The model under review builds one solid part; all positions refer to its coordinate system, in mm. Face numbers are marked on the shaded views. A direction names the side the tool comes from. Coordinates: 2 decimals unless noted, no trailing zeros. Order: outer loops, then holes, each group sorted by start corner. A loop starts at its lowest first (then second) coordinate and runs counter-clockwise, first axis right, second up.
```python
from build123d import *

# Parameters (mm, degrees)
F0_W      = 29
F0_H      = 29
F1_DEPTH  = 42
F2_R      = 14.5
F2_R_2    = 13.5
F3_DEPTH  = 12
F4_W      = 34
F4_H      = 25
F5_DEPTH  = 0.1
F6_W      = 34
F6_H      = 25
F7_DEPTH  = 0.1
F8_W      = 28.9
F8_H      = 34
F9_DEPTH  = 0.1
F11_D     = 3.3
F11_DEPTH = 3
F11_TIP   = 0.9914200214
F13_D     = 2.3
F13_DEPTH = 3
F13_TIP   = 0.6909897119
F14_R     = 6.6
F15_DEPTH = 0.5
F16_W     = 12
F16_H     = 10
F17_DEPTH = 0.5
F19_DEPTH = 10
F20_R     = 5
F20_R_2   = 4.2771578829
F21_DEPTH = 5.8


with BuildPart() as f1:
    # F0 (on Front) → F1 (new body)
    with BuildSketch(Plane.XZ):
        Rectangle(F0_W, F0_H)
    extrude(amount=F1_DEPTH)

    # F2 (on face) → F3 (join)
    with BuildSketch(Plane.XZ.offset(42)):
        Circle(F2_R)
        Circle(F2_R_2, mode=Mode.SUBTRACT)
    extrude(amount=F3_DEPTH)

    # F4 (on face) → F5 (cut)
    with BuildSketch(Plane.YZ.offset(14.5)):
        with Locations((-21, 2)):
            Rectangle(F4_W, F4_H)
    extrude(amount=-F5_DEPTH, mode=Mode.SUBTRACT)

    # F6 (on face) → F7 (cut)
    with BuildSketch(Plane(origin=(-14.5, 0, 0), x_dir=(0, -1, 0), z_dir=(-1, 0, 0))):
        with Locations((21, 2)):
            Rectangle(F6_W, F6_H)
    extrude(amount=-F7_DEPTH, mode=Mode.SUBTRACT)

    # F8 (on face) → F9 (cut)
    with BuildSketch(Plane.XY.offset(14.5)):
        with Locations((0.05, -21)):
            Rectangle(F8_W, F8_H)
    extrude(amount=-F9_DEPTH, mode=Mode.SUBTRACT)

    # F11
    with Locations(Plane(origin=(0, 0, -14.5), x_dir=(1, 0, 0), z_dir=(0, 0, -1))):
        with Locations((0, 15.3), (10, 39), (-10, 39)):
            Hole(F11_D / 2, depth=F11_DEPTH)
            with Locations((0, 0, -(F11_DEPTH + F11_TIP / 2))):  # 118° drill point
                Cone(0, F11_D / 2, F11_TIP, mode=Mode.SUBTRACT)

    # F13
    with Locations(Plane(origin=(0, 0, -14.5), x_dir=(1, 0, 0), z_dir=(0, 0, -1))):
        with Locations((6, 15.5), (-6, 15.5), (6, 37.5), (-6, 37.5)):
            Hole(F13_D / 2, depth=F13_DEPTH)
            with Locations((0, 0, -(F13_DEPTH + F13_TIP / 2))):  # 118° drill point
                Cone(0, F13_D / 2, F13_TIP, mode=Mode.SUBTRACT)

    # F14 (on face) → F15 (join)
    with BuildSketch(Plane(origin=(0, 0, 0), x_dir=(-1, 0, 0), z_dir=(0, 1, 0))):
        with Locations((-7.9, -6.2)):
            Circle(F14_R)
    extrude(amount=F15_DEPTH)

    # F16 (on face) → F17 (cut)
    with BuildSketch(Plane(origin=(0, 0, 0), x_dir=(-1, 0, 0), z_dir=(0, 1, 0))):
        with Locations((2.2, 8.5)):
            Rectangle(F16_W, F16_H)
    extrude(amount=-F17_DEPTH, mode=Mode.SUBTRACT)

    # F18 (on face) → F19 (cut)
    with BuildSketch(Plane(origin=(0, -0.5, 0), x_dir=(-1, 0, 0), z_dir=(0, 1, 0))):
        Polygon((-3.1485289801, 10.3262867779), (-3.1485289801, 4.1849459521), (7.6598110609, 4.1849459521), (7.6598110609, 10.3262867779), (5.341138225, 10.3262867779), (5.341138225, 11.5245990455), (4.3890266679, 11.5245990455), (4.3890266679, 12.9305869341), (0, 12.9305869341), (0, 11.5245990455), (-1.0954904137, 11.5245990455), (-1.0954904137, 10.3262867779), align=None)
    extrude(amount=-F19_DEPTH, mode=Mode.SUBTRACT)

    # F20 (on face) → F21 (join)
    with BuildSketch(Plane(origin=(0, 0.5, 0), x_dir=(-1, 0, 0), z_dir=(0, 1, 0))):
        with Locations((-7.9, -6.2)):
            Circle(F20_R)
        with Locations((-7.9, -6.2)):
            Circle(F20_R_2, mode=Mode.SUBTRACT)
    extrude(amount=F21_DEPTH)


solid = f1.part
```
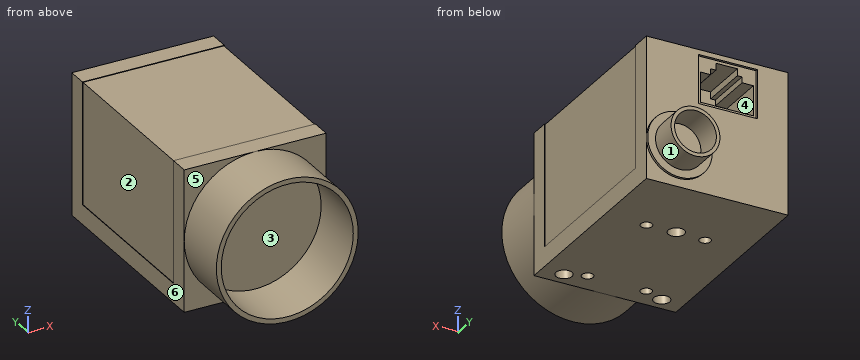
(1) Wall thickness on probe 1 along Y at (x, z) = (6, -12.4); probe 2 along Y at (x, z) = (6, -12.95); probe 3 along X at (y, z) = (-15.3, -12.25): over which ranges is each line inside the solid? List them lowest first.
A:
probe 1: y = -54 to -38.65, -36.35 to -16.65, -14.35 to 0.5
probe 2: y = -54 to -38.65, -36.35 to -16.65, -14.35 to 0
probe 3: x = -14.5 to -7.13, -4.87 to -1.65, 1.65 to 4.87, 7.13 to 14.5
(2) For pin 1 Ø4.5 at (x, z) = (6, 6) entering from -Y; pin 2 Ø10.5 at (x, z) = (5, -8.5) entering from +Y; pin 3 Ø1 at (x, z) = (-10, -5) entering from +Y; pin 4 Ø3 at (x, y) = (6, -15.5) entering from +Z, all flat-tipped, find the tip position at first contact; note any pin that passes through.
A:
pin 1: stops at y = -42
pin 2: stops at y = 6.3
pin 3: stops at y = 0
pin 4: stops at z = 14.4
(3) Draft analysis for pull direction X (two halves, no side actions). For the marked faces 4, 5 and 6, state which applies: released by +X, released by -X, zero draft, split by the parting line, or undercut.
A:
face 4: undercut
face 5: zero draft
face 6: released by -X
(4) We need section B-B, the plane y = -45.5. Write out the cut boundary in (x, z), and give its area (3 significant figures).
A:
outline: circle Ø29 at (0, 0); hole circle Ø27 at (0, 0)
area: 88.0 mm2
(5) Machinability: for the marked faces 1, 2 and 3, which of the approach directions +Z, -Z, +X, -X, +Y, -Y give a long, thin tool a straight path to every point of the face, cutting with its end or side? Answer none if there is none.
A:
face 1: +Y
face 2: +Z, -X
face 3: -Y
(6) We need section A-A, the plane z = 7.25. Write out the cut boundary in (x, y).
A:
outline: (-14.5, -42) - (-12.56, -42) - (-12.56, -54) - (-11.39, -54) - (-11.39, -42) - (11.39, -42) - (11.39, -54) - (12.56, -54) - (12.56, -42) - (14.5, -42) - (14.5, -38) - (14.4, -38) - (14.4, -4) - (14.5, -4) - (14.5, 0) - (3.8, 0) - (3.8, -0.5) - (3.15, -0.5) - (3.15, -10.5) - (-7.66, -10.5) - (-7.66, -0.5) - (-8.2, -0.5) - (-8.2, 0) - (-14.5, 0) - (-14.5, -4) - (-14.4, -4) - (-14.4, -38) - (-14.5, -38) - close
